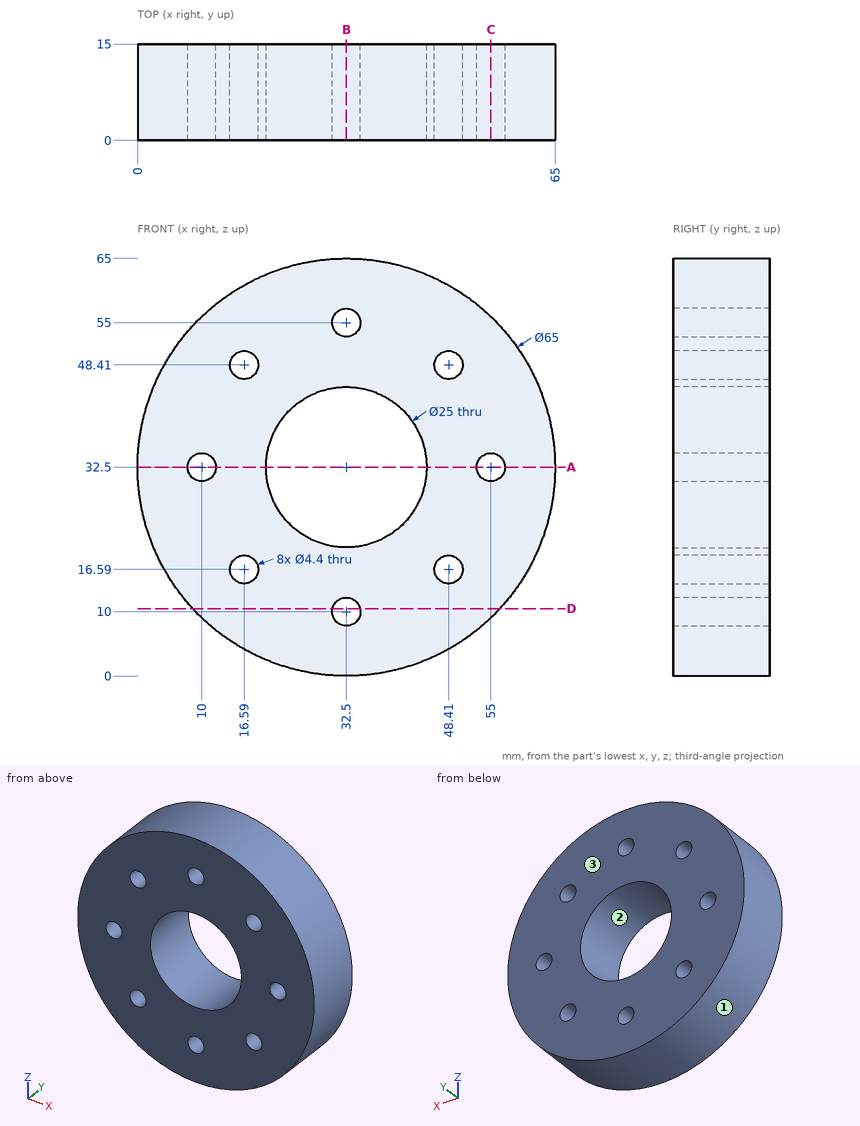
Part print with two shaded views. Sizes in mm from the minimum x, y, z corner. Round coordinates to 2 decimals unless told otherwise and drop trailing zeros. Loops run counter-clockwise (first coordinate to the right, second up) from the corner with the lowest first, then second, coordinate; pieces in that order, holes last. Notation, with made-up numbers: (41.25, -9.75) - (88.25, -9.75) arc R28 ccw to (88.25, 11.25) - close; hole circle Ø1 at (1, 76.5). An arc over 180 degrees is marked (long way). Put each result on its own line as item: value.
1. Two-plate mould, pull along X, no slides. Class the marked faces 1, 2 and 3: released by +X, released by -X, zero draft, split by the parting line, or undercut.
Geometry check:
face 1: split by the parting line
face 2: undercut
face 3: zero draft
2. Slice it at A-A on z = 32.5. List the corners of the cut face in (x, y), and give its area (3 significant figures).
Geometry check:
outline: (0, 0) - (7.8, 0) - (7.8, 15) - (0, 15) - close; (12.2, 0) - (20, 0) - (20, 15) - (12.2, 15) - close; (45, 0) - (52.8, 0) - (52.8, 15) - (45, 15) - close; (57.2, 0) - (65, 0) - (65, 15) - (57.2, 15) - close
area: 468 mm²
3. Slice it at B-B on x = 32.5. List the corners of the cut face in (y, z).
Geometry check:
outline: (0, 0) - (15, 0) - (15, 7.8) - (0, 7.8) - close; (0, 12.2) - (15, 12.2) - (15, 20) - (0, 20) - close; (0, 45) - (15, 45) - (15, 52.8) - (0, 52.8) - close; (0, 57.2) - (15, 57.2) - (15, 65) - (0, 65) - close
4. Slice it at C-C on x = 55. List the corners of the cut face in (y, z).
Geometry check:
outline: (0, 9.05) - (15, 9.05) - (15, 30.3) - (0, 30.3) - close; (0, 34.7) - (15, 34.7) - (15, 55.95) - (0, 55.95) - close
5. Wall check: line 1 (X direction, y = 10, z = 32.5); line 2 (X direction, y = 12.5, z = 15.5); line 3 (Z direction, x = 38.5, y = 14.5). Give the ranges that are in metal, low to high.
Geometry check:
line 1: 0 to 7.8, 12.2 to 20, 45 to 52.8, 57.2 to 65
line 2: 4.8 to 14.68, 18.5 to 46.5, 50.32 to 60.2
line 3: 0.56 to 21.53, 43.47 to 64.44
6. Slice it at D-D on z = 10.5. List the corners of the cut face in (x, y).
Geometry check:
outline: (8.58, 0) - (30.36, 0) - (30.36, 15) - (8.58, 15) - close; (34.64, 0) - (56.42, 0) - (56.42, 15) - (34.64, 15) - close
7. Pin check, flat tips, straight feed: P1, Ø2, axis at y = 5.5, z = 18, coming from the +X side; P2, Ø2, axis at x = 43.5, y = 5.5, coming from the +Z side; P3, Ø3, axis at y = 12, z = 38, coming from the -X side. Stop position of each tip, or through.
Geometry check:
P1: x = 62.06
P2: z = 63.42
P3: x = 0.25
